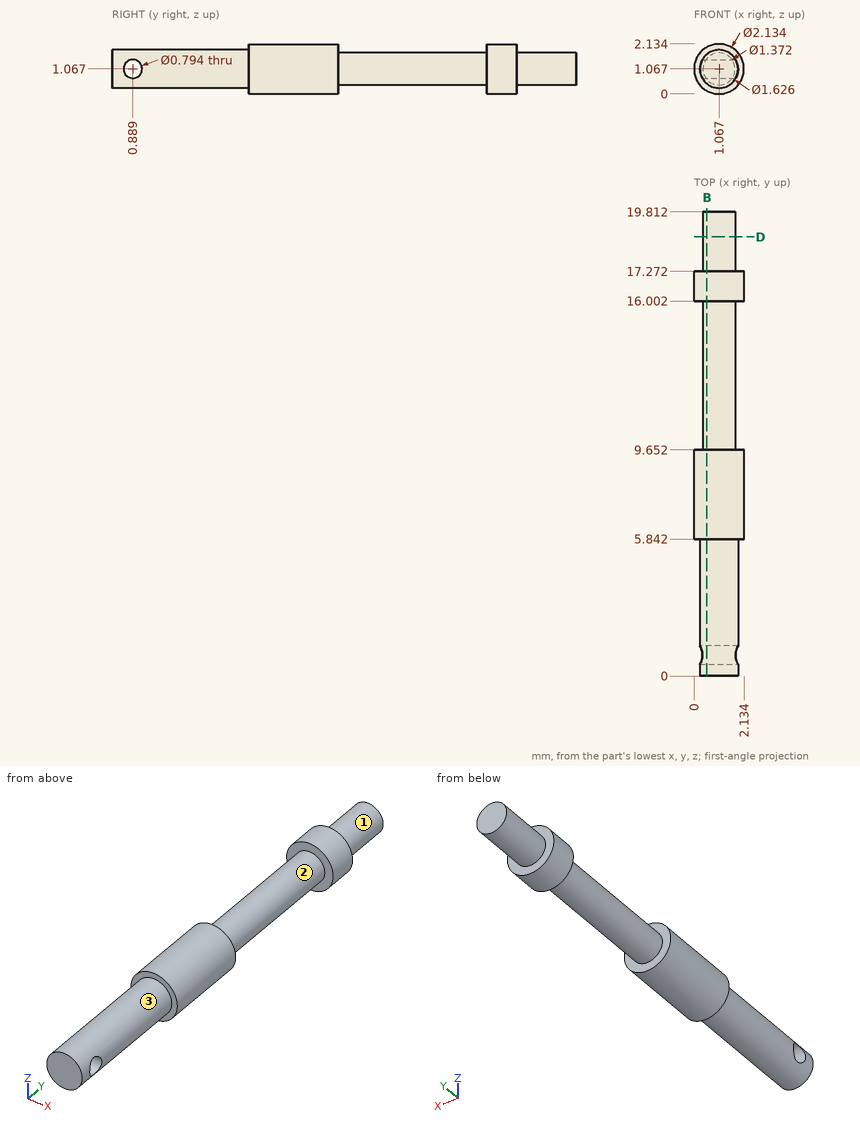
Print and shaded views of the part. All mm, measured from the part's lowest x, y and z. A direction names the side the tool comes from. Give positions to 0.01 mm unless a question says otherwise; leave off trailing zeros. Write each loop counter-clockwise with the first axis right and the second up, starting at its lowest first coordinate (ties: lowest second). Pieces come first, ordered by that corner, then holes. Notation, with made-up numbers: M -27,67.5 L -14,67.5 A25 ccw -14,100.5 Z; hole C 32.25,8 d6. An arc over 180 degrees is marked long. Use a Markdown table: item, result.
1) Tool access for the marked faces 1, 2 and 3: list every direction of +Z, -Z, +X, -X, +Y, -Y with a clear straight run to the whole face (end or side of a thin tool).
Responses:
| item | result |
|---|---|
| face 1 | +Y |
| face 2 | none |
| face 3 | -Y |
2) Cut at B-B (x = 0.55). List the corners of the cut face in (y, z).
Responses:
| item | result |
|---|---|
| outline | M 0,0.44 L 5.84,0.44 L 5.84,0.13 L 9.65,0.13 L 9.65,0.62 L 16,0.62 L 16,0.13 L 17.27,0.13 L 17.27,0.62 L 19.81,0.62 L 19.81,1.52 L 17.27,1.52 L 17.27,2 L 16,2 L 16,1.52 L 9.65,1.52 L 9.65,2 L 5.84,2 L 5.84,1.69 L 0,1.69 Z; hole C 0.89,1.07 d0.79 |
3) Cut at D-D (y = 18.75). List the corners of the cut face in (x, z) (1 decimal).
Responses:
| item | result |
|---|---|
| outline | C 1.1,1.1 d1.4 |
4) Pin check, flat tip, straight feed: pin 1 (1 mm diameter, centred on y = 12, z = 1.5, fed in from -X). Stop position of the tip, or through.
Responses:
| item | result |
|---|---|
| pin 1 | stops at x = 0.38 |
5) Drill centre lines: line 1 (Y direction, x = 1.8, z = 1); line 2 (Y direction, x = 0.55, z = 1.1) (1 decimal); line 3 (Y direction, x = 1.9, z = 0.7). Where is each one in solid material? Low to high. Write a range as from..to.
Responses:
| item | result |
|---|---|
| line 1 | y = 0..0.5, 1.28..9.65, 16..17.27 |
| line 2 | y = 0..0.5, 1.3..19.8 |
| line 3 | y = 5.84..9.65, 16..17.27 |
